The figure shows three views and two pictorial views of one solid part (mm, origin at its lowest corner). Answer the questions. Coordinates: 2 decimals unless noted, no trailing zeros. Loops run counter-clockwise (first coordinate to the right, second up) from the corner with the lowest first, then second, coordinate; pieces in that order, holes last. Notation, with made-up numbers: (-34.5, 10.25) -> (0.5, 10.25) arc R16 ccw to (0.5, 20.25) -> close; hole circle Ø10 at (-26.5, -33). An arc over 180 degrees is marked (long way). Answer as a JSON object with one key per item and string values. Group by question number.
1) Section A-A, the plane z = 5.5 is taken. Count the separate pieces of the cut face and the enclosed holes in it, plus the area to 4 significant figures.
2) Consider probe 1 along X at (y, z) = (299, 17.75); probe 2 along X at (y, z) = (51.5, 4.25); probe 3 along Y at (x, z) = (48, 20.75). Determine where each line is inside the solid, lowest interval first. Write a range as [from, to].
3) Section B-B, the plane y = 210 is taken. Give the vertices of the cut face in (x, z), plus the area to 4 significant figures.
4) Flat-ended cylindrical pins translate along their axes: P1, Ø12.5, axis at y = 11.5, z = 15, coming from the -X side; P2, Ø7.5, axis at x = 790.5, z = 17, coming from the -Y side; P3, Ø12.5, axis at y = 15.5, z = 7, coming from the +X side. Find the tip coordinate at first contact, or state that the pin passes through.
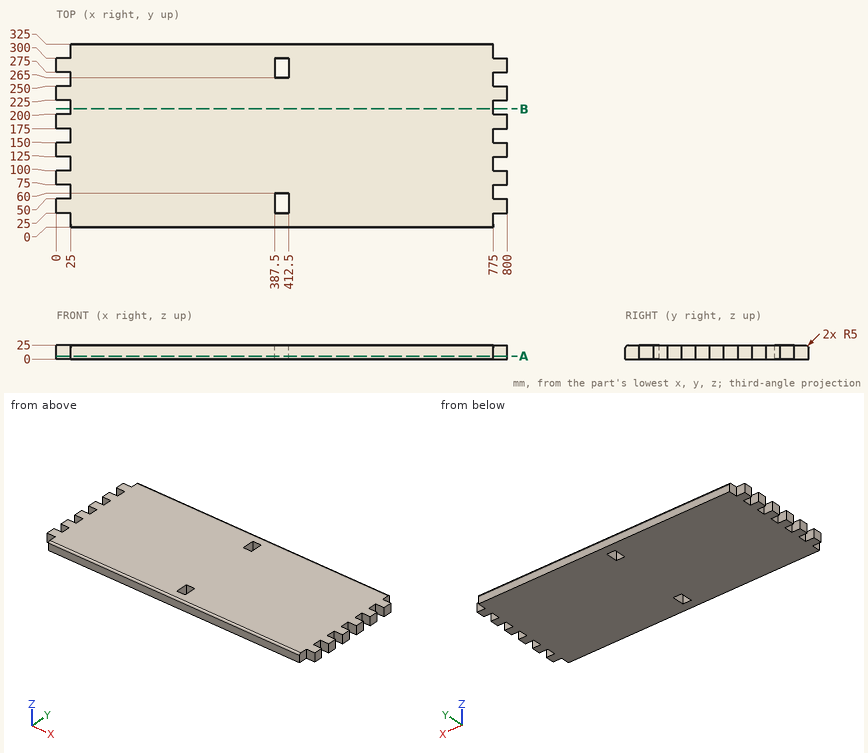
Determined:
{
 "1": {"separate pieces": "1", "enclosed holes": "2", "area": "249,500 mm²"},
 "2": {"probe 1": "[0, 387.5], [412.5, 800]", "probe 2": "[25, 387.5], [412.5, 775]", "probe 3": "[0.06, 324.94]"},
 "3": {"outline": "(25, 0) -> (775, 0) -> (775, 25) -> (25, 25) -> close", "area": "18,750 mm²"},
 "4": {"P1": "x = 25", "P2": "y = 25", "P3": "x = 775"}
}
